Here's the drawing with two shaded views (mm, measured from the low corner). I have some questions. Give positions to 0.01 mm unless a question says otherwise; leave off trailing zeros. Write each loop counter-clockwise with the first axis right and the second up, starting at its lowest first coordinate (ties: lowest second). Pieces come first, ordered by that corner, then holes.
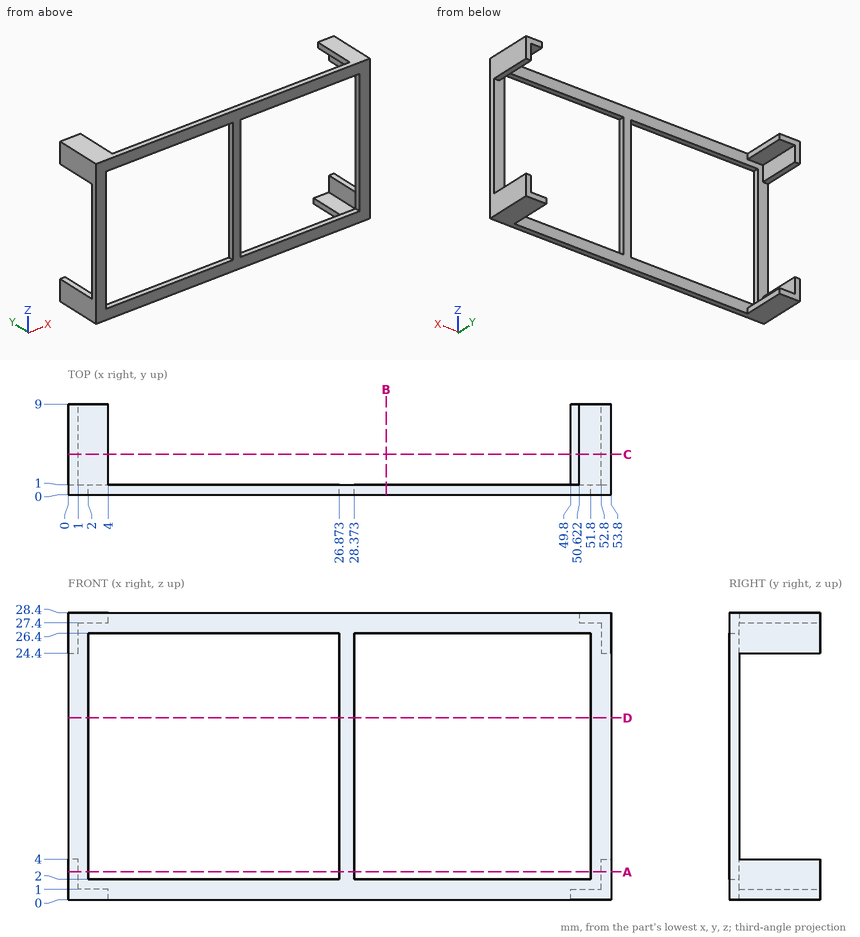
1) Suppose I cut it at C-C on y = 4. Write out the boundary of the cut face in (x, z).
Values follow:
outline: (0, 0) - (4, 0) - (4, 1) - (1, 1) - (1, 4) - (0, 4) - close; (0, 24.4) - (1, 24.4) - (1, 27.4) - (4, 27.4) - (4, 28.4) - (0, 28.4) - close; (49.8, 0) - (53.8, 0) - (53.8, 4) - (52.8, 4) - (52.8, 1) - (49.8, 1) - close; (50.62, 27.4) - (52.8, 27.4) - (52.8, 24.4) - (53.8, 24.4) - (53.8, 28.4) - (50.62, 28.4) - close
2) Suppose I cut it at B-B on x = 31.5. Write out the boundary of the cut face in (y, z).
Values follow:
outline: (0, 0) - (1, 0) - (1, 2) - (0, 2) - close; (0, 26.4) - (1, 26.4) - (1, 28.4) - (0, 28.4) - close
3) Suppose I cut it at D-D on z = 18. Write out the boundary of the cut face in (x, y), plus the area to 3 significant figures.
Values follow:
outline: (0, 0) - (2, 0) - (2, 1) - (0, 1) - close; (26.87, 0) - (28.37, 0) - (28.37, 1) - (26.87, 1) - close; (51.8, 0) - (53.8, 0) - (53.8, 1) - (51.8, 1) - close
area: 5.50 mm2
4) Please list where these lines run through material, in increasing order: L1, parallel to X at y = 0.5, z = 12.5; L2, parallel to X at y = 5.25, z = 25; L3, parallel to Z at x = 51.5, y = 6.25.
Values follow:
L1: x = 0 to 2, 26.87 to 28.37, 51.8 to 53.8
L2: x = 0 to 1, 52.8 to 53.8
L3: z = 0 to 1, 27.4 to 28.4
5) For pin 1 Ø4 at (x, z) = (47.5, 3.5) entering from +Y, with a flat end and sliding along its axis, tell me the tip position at first contact or that it passes through.
Values follow:
pin 1: stops at y = 1
6) Suppose I cut it at A-A on z = 2.75. Write out the boundary of the cut face in (x, y).
Values follow:
outline: (0, 0) - (2, 0) - (2, 1) - (1, 1) - (1, 9) - (0, 9) - close; (26.87, 0) - (28.37, 0) - (28.37, 1) - (26.87, 1) - close; (51.8, 0) - (53.8, 0) - (53.8, 9) - (52.8, 9) - (52.8, 1) - (51.8, 1) - close
